Study the drawing (mm; zero at the part's minimum x, y, z) and answer. A direction names the side the tool comes from. Coordinates: 2 decimals unless noted, no trailing zeros. Order: outer loops, then holes, each group sorted by start corner. A loop starts at its lowest first (then second) coordinate and runs counter-clockwise, first axis right, second up. Notation, with made-up numbers: M 25,39 L 60,39 A27 cw 60,55 Z; hole C -39.5,77.25 d8. An arc over 180 degrees is marked long. One line per item, written item: value. Start each with the question number.
Q1. The part is cut by section C-C on y = 55. Give the vertices of the cut face in (x, z) (1 decimal).
Q2. The part is cut by section D-D on x = 30.5. Give the vertices of the cut face in (y, z) (1 decimal), then the cut area to 3 significant figures.
Q3. Determine the mould class of the marked faces 1, 2 and 3 for opening direction X: pulls with the +X half, pulls with the -X half, needs draft (parallel to the pull), parting line crosses it, or undercut.
Q4. The part is cut by section B-B on z = 69. Give the vertices of the cut face in (x, y), then the cut area to 3 significant figures.
Q5. For the marked faces 4 and 5, determine the directions among +Z, -Z, +X, -X, +Y, -Y from which every point of the face is accessible in a straight line to the end or side of a thin tool.
Q6. Each of these flat-tipped pins is pushed along its axis until it touches: pin 1 Ø1.5 at (y, z) = (25, 49.5) entering from -X; pin 2 Ø1 at (x, y) = (70.5, 23) entering from +Z; pin 3 Ø5 at (x, y) = (49.5, 23.5) entering from -Z. Where does it stop, or does it pass through?
Q7. Straight lines are drawn through the part: line 1 along Y through (x, z) = (32.5, 68); line 2 along Z through (x, y) = (54, 49) (1 decimal); line 3 along Z through (x, y) = (86.5, 11) (1 decimal). For each, find the intervals that lie inside material, in ascending order. Write a range as [from, to].
Q8. The part is cut by section A-A on x = 71. Give the vertices of the cut face in (y, z), then the cut area to 3 significant figures.
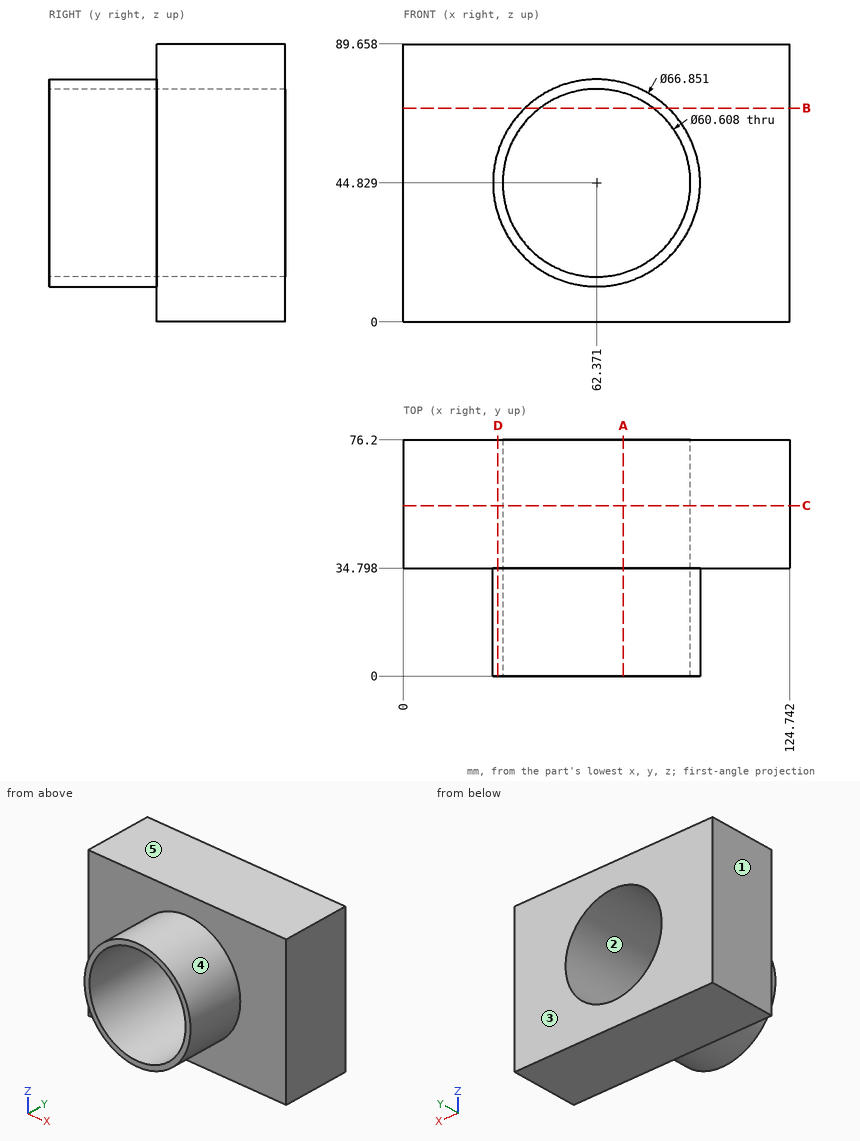
Output:
1. outline: M 0,0 L 124.7,0 L 124.7,89.7 L 0,89.7 Z; hole C 62.4,44.8 d60.6
2. outline: M 0,34.8 L 34.8,34.8 L 34.8,0 L 76.2,0 L 76.2,89.7 L 34.8,89.7 L 34.8,54.9 L 0,54.9 Z
2. area: 4,410 mm^2
3. face 1: pulls with the -X half
3. face 2: undercut
3. face 3: needs draft
4. outline: M 0,34.8 L 39.28,34.8 L 39.28,0 L 44.09,0 L 44.09,76.2 L 0,76.2 Z; M 80.65,0 L 85.46,0 L 85.46,34.8 L 124.74,34.8 L 124.74,76.2 L 80.65,76.2 Z
4. area: 3,990 mm^2
5. face 4: -Y
5. face 5: +Z, +X, -X, +Y, -Y
6. pin 1: stops at x = 29.18
6. pin 2: stops at z = 77.37
6. pin 3: stops at z = 13.05
7. line 1: y = [34.8, 76.2]
7. line 2: z = [0, 15.7], [74, 89.7]
7. line 3: z = [21.7, 26.5], [63.2, 68]
8. outline: M 0,12.54 L 34.8,12.54 L 34.8,0 L 76.2,0 L 76.2,15.78 L 0,15.78 Z; M 0,73.88 L 76.2,73.88 L 76.2,89.66 L 34.8,89.66 L 34.8,77.12 L 0,77.12 Z
8. area: 1,530 mm^2
